Here's how the part is built. I have some questions about the finished solid (model axes, mm). A direction names the side the tool comes from. Round coordinates to 2 decimals unless told otherwise and drop trailing zeros. Order: outer loops, then holes, each group sorted by start corner. A loop starts at its lowest first (then second) coordinate and runs counter-clockwise, first axis right, second up. Notation, with made-up numbers: (-20, 73.25) -> (0, 73.25) arc R16 cw to (0, 78.25) -> close; hole circle Ø6 at (72, 48). An arc over 180 degrees is marked (long way). Use a Markdown table: item, result. Add a question column.
(1) I want a section at A-A, the plane y = 14.5. Please give me the cut outline in (x, z), then the cut area to 3 significant figures.
(2) On a 3-axis mill with a long thin cutter (end or side, diameter ignored), from which of +Z, -Z, +X, -X, +Y, -Y can I reach the whole of each face in a straight line? I mean faces 1 (the face through (4.868, 1.909, 25.454)), 2 (the face through (-12.445, 17.69, -0.07)), 3 (the face through (20, 1, -25)), 4 (the face through (-20, 1, -25)), 5 (the face through (12.4, 2.57, 0.32)). Say none if no direction works.
(3) I want a section at C-C, the plane z = 0. Please give me the cut outline in (x, y), then the cut area to 3 significant figures.
(4) I'm going to push flat-ended pins straight in: P1, Ø12, axis at x = -6, z = -6.5, coming from the +Y side; P2, Ø1.5, axis at x = 5, y = 4, coming from the -Z side; P3, Ø1.5, axis at x = -9, y = 4.5, coming from the -Z side. Where does each tip first touch, or does it pass through?
(5) I want a section at B-B, the plane z = -29.5. Please give me the cut outline in (x, y).
(6) If I drill on probe 1 along Z at (x, y) = (2, 3.75); probe 2 along X at (y, z) = (1, 33); probe 3 along Y at (x, z) = (-13, 34), over which ranges is the centre line in solid material (lowest first)?
(7) Thinking about a two-plate mould opening in X: for faces 6 (the face through (16, 8, 0)), 7 (the face through (14, 15, -5)), 8 (the face through (0, 2, -25)), which applies, pulls with the +X half, pulls with the -X half, needs draft (parallel to the pull), parting line crosses it, or undercut?
from build123d import *

# Parameters (mm, degrees)
SKETCH1_W                = 32
SKETCH1_H                = 50
BOSS_EXTRUDE1_DEPTH      = 5
CUT_EXTRUDE1_DEPTH       = 22.5
BOSS_EXTRUDE2_DEPTH      = 5
BOSS_EXTRUDE3_DEPTH      = 10
BOSS_EXTRUDE3_DEPTH_BACK = 4.5
BOSS_EXTRUDE3_START      = -16
BOSS_EXTRUDE4_START      = 6
BOSS_EXTRUDE4_DEPTH      = 14.5
FILLET1_R                = 2.6
FILLET2_R                = 2.6


with BuildPart() as part:
    # Sketch1 → Boss-Extrude1 (new body)
    with BuildSketch(Plane(origin=(0, 0, 0), x_dir=(1, 0, 0), z_dir=(0, 1, 0))):
        Rectangle(SKETCH1_W, SKETCH1_H)
    extrude(amount=BOSS_EXTRUDE1_DEPTH)

    # Sketch2 → Cut-Extrude1 (cut, symmetric)
    with BuildSketch(Plane.XY):
        with BuildLine():
            Line((-11, 2), (11, 2))
            ThreePointArc((11, 2), (12.414213562, 2.585786438), (13, 4))
            Line((13, 4), (13, 5))
            Line((13, 5), (-13, 5))
            Line((-13, 5), (-13, 4))
            ThreePointArc((-13, 4), (-12.414213562, 2.585786438), (-11, 2))
        make_face()
    extrude(amount=CUT_EXTRUDE1_DEPTH, both=True, mode=Mode.SUBTRACT)

    # Sketch3 → Boss-Extrude2 (add, symmetric)
    with BuildSketch(Plane.XY):
        with BuildLine():
            Line((-16, 5), (-16, 23))
            Line((-16, 23), (-13, 23))
            Line((-13, 23), (-11, 19))
            ThreePointArc((-11, 19), (-12.459649548, 17.666045055), (-13, 15.763932023))
            Line((-13, 15.763932023), (-13, 5))
            Line((-13, 5), (-16, 5))
        make_face()
        with BuildLine():
            Line((16, 5), (13, 5))
            Line((13, 5), (13, 15.763932023))
            ThreePointArc((13, 15.763932023), (12.459649548, 17.666045055), (11, 19))
            Line((11, 19), (13, 23))
            Line((13, 23), (16, 23))
            Line((16, 23), (16, 5))
        make_face()
    extrude(amount=BOSS_EXTRUDE2_DEPTH, both=True)

    # Sketch4 → Boss-Extrude3 (add, two sides: drawn at the far end of the back side and taken through both)
    with BuildSketch(Plane(origin=(0, 0, 0), x_dir=(0, 0, -1), z_dir=(1, 0, 0)).offset(BOSS_EXTRUDE3_START - BOSS_EXTRUDE3_DEPTH_BACK)):
        with BuildLine():
            Line((25, 0), (36.9, 0))
            ThreePointArc((36.9, 0), (37.324264069, 0.175735931), (37.5, 0.6))
            Line((37.5, 0.6), (37.5, 1.8))
            ThreePointArc((37.5, 1.8), (37.324264069, 2.224264069), (36.9, 2.4))
            Line((36.9, 2.4), (25, 2.4))
            Line((25, 2.4), (25, 0))
        make_face()
        with BuildLine():
            Line((-25, 0), (-36.9, 0))
            ThreePointArc((-36.9, 0), (-37.324264069, 0.175735931), (-37.5, 0.6))
            Line((-37.5, 0.6), (-37.5, 1.8))
            ThreePointArc((-37.5, 1.8), (-37.324264069, 2.224264069), (-36.9, 2.4))
            Line((-36.9, 2.4), (-25, 2.4))
            Line((-25, 2.4), (-25, 0))
        make_face()
    extrude(amount=BOSS_EXTRUDE3_DEPTH + BOSS_EXTRUDE3_DEPTH_BACK)

    # Sketch4<2> → Boss-Extrude4 (add)
    with BuildSketch(Plane(origin=(0, 0, 0), x_dir=(0, 0, -1), z_dir=(1, 0, 0)).offset(BOSS_EXTRUDE4_START)):
        with BuildLine():
            Line((25, 0), (36.9, 0))
            ThreePointArc((36.9, 0), (37.324264069, 0.175735931), (37.5, 0.6))
            Line((37.5, 0.6), (37.5, 1.8))
            ThreePointArc((37.5, 1.8), (37.324264069, 2.224264069), (36.9, 2.4))
            Line((36.9, 2.4), (25, 2.4))
            Line((25, 2.4), (25, 0))
        make_face()
        with BuildLine():
            Line((-25, 0), (-36.9, 0))
            ThreePointArc((-36.9, 0), (-37.324264069, 0.175735931), (-37.5, 0.6))
            Line((-37.5, 0.6), (-37.5, 1.8))
            ThreePointArc((-37.5, 1.8), (-37.324264069, 2.224264069), (-36.9, 2.4))
            Line((-36.9, 2.4), (-25, 2.4))
            Line((-25, 2.4), (-25, 0))
        make_face()
    extrude(amount=BOSS_EXTRUDE4_DEPTH)

    # Fillet1
    fillet1_edges = [part.edges().sort_by_distance(p)[0] for p in [
        (-14.5, 5, 5),
        (14.5, 5, 5),
        (-14.5, 5, -5),
        (14.5, 5, -5),
        (-6, 1.2, -25),
        (6, 1.2, -25),
        (6, 1.2, 25),
        (-6, 1.2, 25),
        (-11, 2.4, -25),
        (11, 2.4, -25),
        (-11, 2.4, 25),
        (11, 2.4, 25),
    ]]
    fillet(fillet1_edges, radius=FILLET1_R - 0.0001)  # a hair under: the kernel refuses the full size

    # Fillet2
    fillet2_edges = [part.edges().sort_by_distance(p)[0] for p in [
        (-16, 2.4, 26.29995),
        (-16, 2.4, -26.29995),
        (-16, 1.2, 25),
        (-16, 1.2, -25),
        (16, 1.2, -25),
        (16, 2.4, -26.29995),
        (16, 2.4, 26.29995),
        (16, 1.2, 25),
    ]]
    fillet(fillet2_edges, radius=FILLET2_R - 0.0004)  # a hair under: the kernel refuses the full size


solid = part.part
Taken from the geometry:
| question | item | result |
|---|---|---|
| 1 | outline | (-16, -5) -> (-13, -5) -> (-13, 5) -> (-16, 5) -> close; (13, -5) -> (16, -5) -> (16, 5) -> (13, 5) -> close |
| 1 | area | 60.0 mm2 |
| 2 | face 1 | +Z, +Y, -Y |
| 2 | face 2 | +Z, -Z |
| 2 | face 3 | +X, +Y, -Y |
| 2 | face 4 | -X, +Y, -Y |
| 2 | face 5 | none |
| 3 | outline | (-16, 0) -> (16, 0) -> (16, 23) -> (13, 23) -> (11, 19) arc R3.62 cw to (13, 15.76) -> (13, 4) arc R2 cw to (11, 2) -> (-11, 2) arc R2 cw to (-13, 4) -> (-13, 15.76) arc R3.62 cw to (-11, 19) -> (-13, 23) -> (-16, 23) -> close |
| 3 | area | 203 mm2 |
| 4 | P1 | stops at y = 20.62 |
| 4 | P2 | stops at z = -25.67 |
| 4 | P3 | stops at z = -25.32 |
| 5 | outline | (-20.5, 0) -> (-6, 0) -> (-6, 2.4) -> (-20.5, 2.4) -> close; (6, 0) -> (20.5, 0) -> (20.5, 2.4) -> (6, 2.4) -> close |
| 6 | probe 1 | z = -25 to -22.5, 22.5 to 25 |
| 6 | probe 2 | x = -20.5 to -6, 6 to 20.5 |
| 6 | probe 3 | y = 0 to 2.4 |
| 7 | face 6 | pulls with the +X half |
| 7 | face 7 | needs draft |
| 7 | face 8 | undercut |
